Here's how the part is built. I have some questions about the finished solid (model axes, mm). Face numbers are marked on the shaded views. A direction names the side the tool comes from. Give positions to 0.01 mm unless a question says otherwise; leave off trailing zeros. Write each loop counter-clockwise with the first axis right and the second up, starting at its lowest first coordinate (ties: lowest second). Pieces come first, ordered by that corner, then holes. Notation, with made-up numbers: (67, 46) -> (110, 46) arc R20 ccw to (110, 56) -> close; hole circle Ø7 at (69.5, 64). An arc over 180 degrees is marked (long way). Answer as CSV lines item,"result". Start each with the question number.
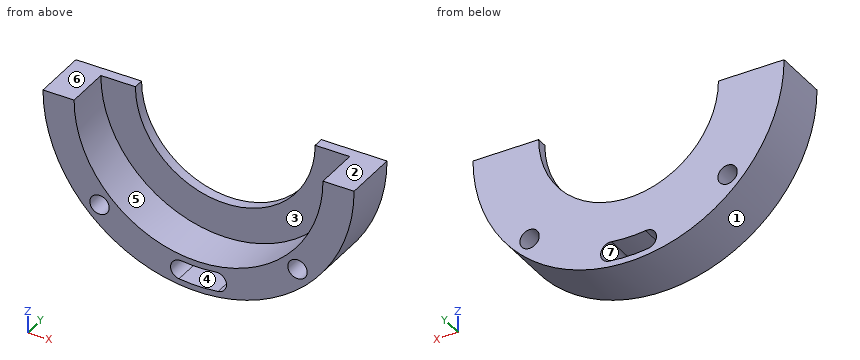
from build123d import *

# Parameters (mm, degrees)
SKETCH1_R           = 28.575
BOSS_EXTRUDE1_DEPTH = 10.16
SKETCH2_R           = 16.51
CUT_EXTRUDE1_DEPTH  = 42.66877548
SKETCH3_R           = 22.86
CUT_EXTRUDE2_DEPTH  = 8.255
SKETCH4_W           = 88.915115744
SKETCH4_H           = 51.352535237
CUT_EXTRUDE3_DEPTH  = 42.66877548
CUT_EXTRUDE4_REACH  = 43.669
SKETCH6_R           = 1.778
CUT_EXTRUDE5_DEPTH  = 42.66877548


with BuildPart() as part:
    # Sketch1 → Boss-Extrude1 (new body)
    with BuildSketch(Plane(origin=(0, 0, 0), x_dir=(1, 0, 0), z_dir=(0, 1, 0))):
        with Locations(Location((0, 0, 0), (0, 0, 270))):
            Circle(SKETCH1_R)
    extrude(amount=BOSS_EXTRUDE1_DEPTH)

    # Sketch2 → Cut-Extrude1 (cut, through all)
    with BuildSketch(Plane.XZ):
        with Locations(Location((0, 0, 0), (0, 0, 270))):
            Circle(SKETCH2_R)
    extrude(amount=-CUT_EXTRUDE1_DEPTH, mode=Mode.SUBTRACT)

    # Sketch3 → Cut-Extrude2 (cut)
    with BuildSketch(Plane.XZ):
        with Locations(Location((0, 0, 0), (0, 0, 270))):
            Circle(SKETCH3_R)
    extrude(amount=-CUT_EXTRUDE2_DEPTH, mode=Mode.SUBTRACT)

    # Sketch4 → Cut-Extrude3 (cut, through all)
    with BuildSketch(Plane(origin=(0, 10.16, 0), x_dir=(1, 0, 0), z_dir=(0, 1, 0))):
        with Locations((4.883047594, -25.676267619)):
            Rectangle(SKETCH4_W, SKETCH4_H)
    extrude(amount=-CUT_EXTRUDE3_DEPTH, mode=Mode.SUBTRACT)

    # Sketch6 → Cut-Extrude4 (cut, up to next)
    with BuildSketch(Plane.XZ, mode=Mode.PRIVATE) as cut_extrude4_sk1:
        with Locations(Location((18.185018645, -18.185018645, 0), (0, 0, 270))):
            Circle(SKETCH6_R)
    cut_extrude4_tool1 = extrude(cut_extrude4_sk1.sketch, amount=-CUT_EXTRUDE4_REACH, mode=Mode.PRIVATE) & part.part
    # Sketch6 → Cut-Extrude4 (cut, up to next)
    with BuildSketch(Plane.XZ, mode=Mode.PRIVATE) as cut_extrude4_sk2:
        with Locations(Location((-18.185018645, -18.185018645, 0), (0, 0, 270))):
            Circle(SKETCH6_R)
    cut_extrude4_tool2 = extrude(cut_extrude4_sk2.sketch, amount=-CUT_EXTRUDE4_REACH, mode=Mode.PRIVATE) & part.part
    add(cut_extrude4_tool1.solids().sort_by_distance((18.185019, 0, -18.185019))[0], mode=Mode.SUBTRACT)
    add(cut_extrude4_tool2.solids().sort_by_distance((-18.185019, 0, -18.185019))[0], mode=Mode.SUBTRACT)

    # Sketch7 → Cut-Extrude5 (cut, through all)
    with BuildSketch(Plane(origin=(0, 10.16, 0), x_dir=(1, 0, 0), z_dir=(0, 1, 0))):
        with BuildLine():
            ThreePointArc((3.124731779, 23.734694259), (0, 23.9395), (-3.124731779, 23.734694259))
            ThreePointArc((-3.124731779, 23.734694259), (-5.119596312, 25.265407653), (-3.588882918, 27.260272186))
            ThreePointArc((-3.588882918, 27.260272186), (0, 27.4955), (3.588882918, 27.260272186))
            ThreePointArc((3.588882918, 27.260272186), (5.119596312, 25.265407653), (3.124731779, 23.734694259))
        make_face()
    extrude(amount=-CUT_EXTRUDE5_DEPTH, mode=Mode.SUBTRACT)


solid = part.part
Item 1: If I drill on line 1 (X direction, y = 4.5, z = -18); line 2 (X direction, y = 8.5, z = -19.75); line 3 (Y direction, x = -3, z = -17.5) (3 decimals), over which ranges is the centre line in solid material (lowest first)? Write a range as [from, to].
Item 2: If we section it at D-D (y = 5.75): State how many separate pieces and enclosed holes the cut face has, and give its area (3 significant figures).
Item 3: I'm going to push flat-ended pins straight in: pin 1 (4.5 mm diameter, centred on x = -18.19, z = -18.19, fed in from -Y); pin 2 (6 mm diameter, centred on x = 9.5, z = -6.5, fed in from -Y); pin 3 (2 mm diameter, centred on x = 22, y = 8, fed in from -Z); pin 4 (4 mm diameter, centred on y = 2, z = -18, fed in from +X). Where does each tip first touch, or does it pass through?
Item 4: If we section it at B-B (z = -24.75): Please give me the cut outline in (x, y).
Item 5: If we section it at C-C (z = -18): Please give me the cut outline in (x, y) (3 decimals), and give its area (3 significant figures).
Item 6: We'd pull the mould along X, two halves only. Please class the marked faces 1, 2, 3 and 4: released by +X, released by -X, zero draft, split by the parting line, or undercut.
Item 7: If we section it at A-A (x = 0): Please give me the cut outline in (y, z) (1 decimal), and give its area (3 significant figures).
Item 8: For the marked faces 5, 6 and 7, which set-ups out of +Z, -Z, +X, -X, +Y, -Y let a thin tool reach every point of the face, with its end or its side?
Final values:
1,line 1,"[-22.19, -19.95], [-16.42, -14.09], [14.09, 16.42], [19.95, 22.19]"
1,line 2,"[-20.65, -19.03], [-17.34, 17.34], [19.03, 20.65]"
1,line 3,"[8.255, 10.16]"
2,separate pieces,"1"
2,enclosed holes,"3"
2,area,"408 mm2"
3,pin 1,"y = 0"
3,pin 2,"through"
3,pin 3,"z = -19.38"
3,pin 4,"x = 23.68"
4,outline,"(-14.28, 0) -> (-4.97, 0) -> (-4.97, 10.16) -> (-14.28, 10.16) -> close; (4.97, 0) -> (14.28, 0) -> (14.28, 10.16) -> (4.97, 10.16) -> close"
5,outline,"(-22.193, 0) -> (-19.953, 0) -> (-19.953, 10.16) -> (-22.193, 10.16) -> close; (-16.417, 0) -> (-14.092, 0) -> (-14.092, 8.255) -> (14.092, 8.255) -> (14.092, 0) -> (16.417, 0) -> (16.417, 10.16) -> (-16.417, 10.16) -> close; (19.953, 0) -> (22.193, 0) -> (22.193, 10.16) -> (19.953, 10.16) -> close"
5,area,"146 mm2"
6,face 1,"split by the parting line"
6,face 2,"zero draft"
6,face 3,"undercut"
6,face 4,"undercut"
7,outline,"(0, -28.6) -> (10.2, -28.6) -> (10.2, -27.5) -> (0, -27.5) -> close; (0, -23.9) -> (10.2, -23.9) -> (10.2, -16.5) -> (8.3, -16.5) -> (8.3, -22.9) -> (0, -22.9) -> close"
7,area,"34.0 mm2"
8,face 5,"+Z, -Y"
8,face 6,"+Z, +X, -X, +Y, -Y"
8,face 7,"+Y, -Y"
